from build123d import *

# Parameters (mm, degrees)
SCHIZZO1_W                   = 58
SCHIZZO1_H                   = 121
ESTRUSIONE_ESTRUSIONE2_DEPTH = 5
TAGLIO_ESTRUSIONE1_REACH     = 7
SCHIZZO12_R                  = 1.6
SCHIZZO2_R                   = 3
ESTRUSIONE_ESTRUSIONE3_DEPTH = 55
RACCORDO1_R                  = 2
FORO_PER_VITE_M3_1_D         = 2.4
FORO_PER_VITE_M3_1_DEPTH     = 20
FORO_PER_VITE_M3_1_TIP       = 0.721032743


with BuildPart() as part:
    # Schizzo1 → Estrusione-Estrusione2 (new body)
    with BuildSketch(Plane.XY):
        with Locations((115.836484846, -73.380424615)):
            Rectangle(SCHIZZO1_W, SCHIZZO1_H)
    extrude(amount=ESTRUSIONE_ESTRUSIONE2_DEPTH)

    # Schizzo12 → Taglio-Estrusione1 (cut, up to next)
    with BuildSketch(Plane(origin=(0, 0, 0), x_dir=(-1, 0, 0), z_dir=(0, 0, -1)), mode=Mode.PRIVATE) as taglio_estrusione1_sk1:
        with Locations((-94.836484846, -102.380424615)):
            Circle(SCHIZZO12_R)
    taglio_estrusione1_tool1 = extrude(taglio_estrusione1_sk1.sketch, amount=-TAGLIO_ESTRUSIONE1_REACH, mode=Mode.PRIVATE) & part.part
    add(taglio_estrusione1_tool1.solids().sort_by_distance((94.836485, -102.380425, 0))[0], mode=Mode.SUBTRACT)
    # Schizzo12 → Taglio-Estrusione1 (cut, up to next)
    with BuildSketch(Plane(origin=(0, 0, 0), x_dir=(-1, 0, 0), z_dir=(0, 0, -1)), mode=Mode.PRIVATE) as taglio_estrusione1_sk2:
        with Locations((-136.836484846, -102.380424615)):
            Circle(SCHIZZO12_R)
    taglio_estrusione1_tool2 = extrude(taglio_estrusione1_sk2.sketch, amount=-TAGLIO_ESTRUSIONE1_REACH, mode=Mode.PRIVATE) & part.part
    add(taglio_estrusione1_tool2.solids().sort_by_distance((136.836485, -102.380425, 0))[0], mode=Mode.SUBTRACT)
    # Schizzo12 → Taglio-Estrusione1 (cut, up to next)
    with BuildSketch(Plane(origin=(0, 0, 0), x_dir=(-1, 0, 0), z_dir=(0, 0, -1)), mode=Mode.PRIVATE) as taglio_estrusione1_sk3:
        with Locations((-136.836484846, -23.380424615)):
            Circle(SCHIZZO12_R)
    taglio_estrusione1_tool3 = extrude(taglio_estrusione1_sk3.sketch, amount=-TAGLIO_ESTRUSIONE1_REACH, mode=Mode.PRIVATE) & part.part
    add(taglio_estrusione1_tool3.solids().sort_by_distance((136.836485, -23.380425, 0))[0], mode=Mode.SUBTRACT)
    # Schizzo12 → Taglio-Estrusione1 (cut, up to next)
    with BuildSketch(Plane(origin=(0, 0, 0), x_dir=(-1, 0, 0), z_dir=(0, 0, -1)), mode=Mode.PRIVATE) as taglio_estrusione1_sk4:
        with Locations((-94.836484846, -23.380424615)):
            Circle(SCHIZZO12_R)
    taglio_estrusione1_tool4 = extrude(taglio_estrusione1_sk4.sketch, amount=-TAGLIO_ESTRUSIONE1_REACH, mode=Mode.PRIVATE) & part.part
    add(taglio_estrusione1_tool4.solids().sort_by_distance((94.836485, -23.380425, 0))[0], mode=Mode.SUBTRACT)

    # Schizzo2 → Estrusione-Estrusione3 (add)
    with BuildSketch(Plane.XY.offset(5)):
        with Locations((140.336484846, -129.380424615)):
            Circle(SCHIZZO2_R)
        with Locations((91.336484846, -129.380424615)):
            Circle(SCHIZZO2_R)
        with Locations((140.336484846, -17.380424615)):
            Circle(SCHIZZO2_R)
        with Locations((91.336484846, -17.380424615)):
            Circle(SCHIZZO2_R)
    extrude(amount=ESTRUSIONE_ESTRUSIONE3_DEPTH)

    # Raccordo1
    raccordo1_edges = [part.edges().sort_by_distance(p)[0] for p in [
        (88.336484846, -129.380424615, 5),
        (137.336484846, -17.380424615, 5),
        (137.336484846, -129.380424615, 5),
        (88.336484846, -17.380424615, 5),
    ]]
    fillet(raccordo1_edges, radius=RACCORDO1_R)

    # Foro per Vite M3-1
    with Locations(Plane.XY.offset(60)):
        with Locations((140.336484846, -129.380424615), (91.336484846, -129.380424615), (91.336484846, -17.380424615), (140.336484846, -17.380424615)):
            Hole(FORO_PER_VITE_M3_1_D / 2, depth=FORO_PER_VITE_M3_1_DEPTH)
            with Locations((0, 0, -(FORO_PER_VITE_M3_1_DEPTH + FORO_PER_VITE_M3_1_TIP / 2))):  # 118° drill point
                Cone(0, FORO_PER_VITE_M3_1_D / 2, FORO_PER_VITE_M3_1_TIP, mode=Mode.SUBTRACT)


solid = part.part
For this review, take the finished solid that the model builds, in its own axes (mm). A direction names the side the tool comes from. Coordinates: 2 decimals unless noted, no trailing zeros. Loops run counter-clockwise (first coordinate to the right, second up) from the corner with the lowest first, then second, coordinate; pieces in that order, holes last. Notation, with made-up numbers: (-12.75, -6.75) -> (9.25, -6.75) arc R18 cw to (9.25, 3.25) -> close; hole circle Ø10 at (-29.75, 44.25). An arc over 180 degrees is marked (long way). Write each question's results on one line, items separated by ' | '.
Q1. Add section D-D, the plane y = -39.5. State the section outline as (x, z) points.
Taken from the geometry:
outline: (86.84, 0) -> (144.84, 0) -> (144.84, 5) -> (86.84, 5) -> close
Q2. Machinability: for faces 1 (the flat face through (87, -14, 5)), 2 (the flat face through (140, -131, 60)), 3 (the cylindrical face through (88.96, -19.21, 33.09)), which of the approach directions +Z, -Z, +X, -X, +Y, -Y give a long, thin tool a straight path to every point of the face, cutting with its end or side? Answer none if there is none.
Taken from the geometry:
face 1: +Z, -X, +Y | face 2: +Z, +X, -X, +Y, -Y | face 3: +Z
Q3. For pin 1 Ø3.5 at (x, y) = (94.84, -102.38) entering from +Z; pin 2 Ø1.2 at (x, y) = (87.5, -14) entering from +Z; pin 3 Ø1.2 at (x, y) = (144, -132.5) entering from +Z; pin 4 Ø2 at (x, z) = (121, 7) entering from +Y, all flat-tipped, find the tip position at first contact; note any pin that passes through.
Taken from the geometry:
pin 1: z = 5 | pin 2: z = 5.06 | pin 3: z = 5.16 | pin 4: through
Q4. Mouldability with a two-part tool opening along Y and no side actions: class faces 4 (the flat face through (115, -133.88, 2)), 5 (the cylindrical face through (90.946, -126.406, 33.085)), 6 (the flat face through (144, -133, 5)) as +Y half, -Y half, draft (parallel to the pull), parting line (faces both ways), or undercut.
Taken from the geometry:
face 4: -Y half | face 5: undercut | face 6: draft
Q5. Add section C-C, the plane x = 120. State the section outline as (y, z) points, then the cut area to 3 significant figures.
Taken from the geometry:
outline: (-133.88, 0) -> (-12.88, 0) -> (-12.88, 5) -> (-133.88, 5) -> close | area: 605 mm²
Q6. Add section B-B, the plane z = 18. State the section outline as (x, y) points, then the cut area to 3 significant figures.
Taken from the geometry:
outline: circle Ø6 at (91.34, -129.38); circle Ø6 at (91.34, -17.38); circle Ø6 at (140.34, -129.38); circle Ø6 at (140.34, -17.38) | area: 113 mm²
Q7. Add section A-A, the plane z = 43.5. State the section outline as (x, y) points.
Taken from the geometry:
outline: circle Ø6 at (91.34, -129.38); circle Ø6 at (91.34, -17.38); circle Ø6 at (140.34, -129.38); circle Ø6 at (140.34, -17.38); hole circle Ø2.4 at (91.34, -129.38); hole circle Ø2.4 at (91.34, -17.38); hole circle Ø2.4 at (140.34, -129.38); hole circle Ø2.4 at (140.34, -17.38)
Q8. To check wall thickness, follow line 1 along Z through (x, y) = (124.5, -114); line 2 along Y through (x, z) = (141, 33.5); line 3 along Z through (x, y) = (93.5, -20). State the ranges of each line that lie inside material, in increasing order. Write a range as [from, to].
Taken from the geometry:
line 1: [0, 5] | line 2: [-132.31, -126.45], [-20.31, -14.45] | line 3: [0, 5.8]
